Read the model definition and answer for the solid it produces. Units are mm, in the model's axes. A direction names the side the tool comes from. Round coordinates to 2 decimals unless told otherwise and drop trailing zeros. Loops run counter-clockwise (first coordinate to the right, second up) from the corner with the lowest first, then second, coordinate; pieces in that order, holes last. Notation, with made-up numbers: (47, 17.25) - (67, 17.25) arc R31 cw to (67, 55.25) - close; hole circle Ø4 at (-23.5, -6). An arc over 180 degrees is marked (long way). Use one line per item in the form item = value. Start each with the question number.
```python
from build123d import *

# Parameters (mm, degrees)
CHAMFER1_SIZE = 0.635
SKETCH3_W     = 0.6731
SKETCH3_H     = 1.1684
FILLET1_R     = 0.396875


with BuildPart() as part:
    # Sketch1 → Revolve1 (revolve)
    with BuildSketch(Plane.XY, mode=Mode.PRIVATE) as revolve1_sk:
        Polygon((-19.05, 50.4825), (-19.05, 46.0375), (-11.8999, 46.0375), (-11.8999, 30.7975), (-11.0998, 30.7975), (-11.0998, 0), (-9.5885, 0), (-9.5885, 50.4825), align=None)
    revolve(revolve1_sk.sketch.rotate(Axis((0, 18.282782329, 0), (0, -1, 0)), 270), axis=Axis((0, 18.282782329, 0), (0, -1, 0)))  # turned: the seam where the file's is

    # Chamfer1
    chamfer1_edges = [part.edges().sort_by_distance(p)[0] for p in [
        (0, 0, -11.0998),
    ]]
    chamfer(chamfer1_edges, length=CHAMFER1_SIZE)

    # Sketch3 → Cut-Revolve1 (revolve, cut)
    with BuildSketch(Plane.XY, mode=Mode.PRIVATE) as cut_revolve1_sk:
        with Locations((-10.76325, 3.7592)):
            Rectangle(SKETCH3_W, SKETCH3_H)
    revolve(cut_revolve1_sk.sketch.rotate(Axis((0, -2.070057214, 0), (0, 1, 0)), 90), axis=Axis((0, -2.070057214, 0), (0, 1, 0)), mode=Mode.SUBTRACT)  # turned: the seam where the file's is

    # Fillet1
    fillet1_edges = [part.edges().sort_by_distance(p)[0] for p in [
        (0, 46.0375, -11.8999),
        (0, 30.7975, -11.0998),
    ]]
    fillet(fillet1_edges, radius=FILLET1_R)


solid = part.part
```
1) A cutting plane is placed at C-C on y = 10. Write down the section's boundary in (x, z), plus the area to 3 significant figures.
2) Straight lines are drawn through the part: line 1 (X direction, y = 15, z = 0); line 2 (X direction, y = 40, z = 0); line 3 (Y direction, x = -7, z = -12.5). For each, find the intervals that lie inside material, in ascending order. Write a range as from..to.
3) For faces 4 (the cylindrical face through (-10.18, 3.77, -2.26)), 5 (the cylindrical face through (11.59, 48.23, -15.12)), 6 (the flat face through (12, 46.038, 4)), determine the directions among +Z, -Z, +X, -X, +Y, -Y from which every point of the face is accessible in a straight line to the end or side of a thin tool.
4) A cutting plane is placed at D-D on y = 32. Write down the section's boundary in (x, z).
5) Flat-ended cylindrical pins translate along their axes: pin 1 (11 mm diameter, centred on x = 0.5, z = -3.5, fed in from +Y); pin 2 (12 mm diameter, centred on x = -4.5, y = 19, fed in from +Z); pin 3 (8 mm diameter, centred on y = 34.5, z = 1, fed in from +X); pin 4 (2 mm diameter, centred on x = -14, z = -4, fed in from -Y). Find the tip coordinate at first contact, or state that the pin passes through.
6) Determine the mould class of faces 1 (the flat face through (-8, 4.343, 7)), 2 (the cylindrical face through (4.251, 1.887, 10.253)), 3 (the cylindrical face through (-9.507, 25.595, -1.248)) for opening direction Z: +Z half, -Z half, draft (parallel to the pull), parting line (faces both ways), or undercut.
Checks:
q1.outline = circle Ø22.2 at (0, 0); hole circle Ø19.18 at (0, 0)
q1.area = 98.2 mm²
q2.line_1 = -11.1..-9.59, 9.59..11.1
q2.line_2 = -11.9..-9.59, 9.59..11.9
q2.line_3 = 46.04..50.48
q3.face_4 = none
q3.face_5 = +Y, -Y
q3.face_6 = -Y
q4.outline = circle Ø23.8 at (0, 0); hole circle Ø19.18 at (0, 0)
q5.pin_1 = through
q5.pin_2 = 11.1
q5.pin_3 = 11.9
q5.pin_4 = 46.04
q6.face_1 = draft
q6.face_2 = parting line
q6.face_3 = undercut
